Read the model definition and answer for the solid it produces. Units are mm, in the model's axes. Face numbers are marked on the shaded views. Give positions to 0.01 mm unless a question says otherwise; leave off trailing zeros. Order: outer loops, then holes, each group sorted by start corner. A loop starts at its lowest first (then second) coordinate and runs counter-clockwise, first axis right, second up. Notation, with made-up numbers: (59, 48.5) - (65, 48.5) arc R23 cw to (65, 61.5) - close; hole circle Ø5 at (-20.5, 16.25). An arc over 180 degrees is marked (long way). Answer as CSV lines item,"result". Start each with the question number.
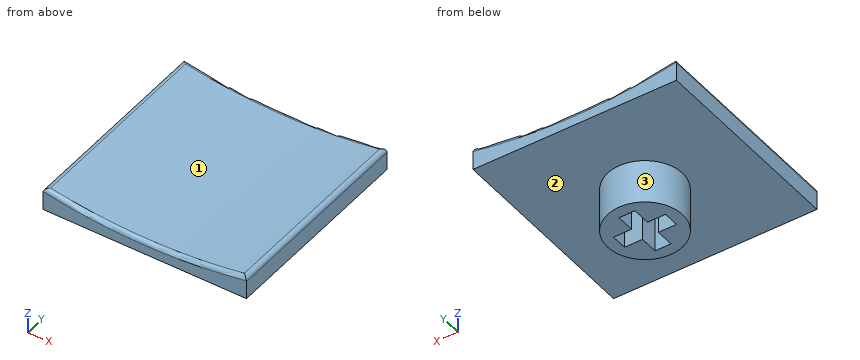
from build123d import *

# Parameters (mm, degrees)
SKETCH_W       = 15.24
SKETCH_H       = 15.24
PAD_DEPTH      = 2
CYLINDER_R     = 40
CYLINDER_DEPTH = 18
FILLET_R       = 0.3
SKETCH001_R    = 2.8
PAD001_DEPTH   = 3.3
POCKET_DEPTH   = 3.3


with BuildPart() as part:
    # Sketch → Pad (new body)
    with BuildSketch(Plane.XY):
        Rectangle(SKETCH_W, SKETCH_H)
    extrude(amount=PAD_DEPTH)

    # Cylinder → Cylinder (cut)
    with BuildSketch(Plane(origin=(0, 9, 41), x_dir=(1, 0, 0), z_dir=(0, -1, 0))):
        Circle(CYLINDER_R)
    extrude(amount=CYLINDER_DEPTH, mode=Mode.SUBTRACT)

    # Fillet
    fillet_edges = [part.edges().sort_by_distance(p)[0] for p in [
        (0, -7.62, 1),
        (-7.62, 0, 1.732512),
        (7.62, 0, 1.732512),
        (0, 7.62, 1),
    ]]
    fillet(fillet_edges, radius=FILLET_R)

    # Sketch001 (on Face4 of Fillet) → Pad001 (join)
    with BuildSketch(Plane(origin=(0, 9, 0), x_dir=(1, 0, 0), z_dir=(0, 0, -1))):
        with Locations((0, 9)):
            Circle(SKETCH001_R)
    extrude(amount=PAD001_DEPTH)

    # Sketch002 (on Face12 of Pad001) → Pocket (cut)
    with BuildSketch(Plane(origin=(0, 9, -3.3), x_dir=(1, 0, 0), z_dir=(0, 0, -1))):
        Polygon((-0.595, 10.95), (0.595, 10.95), (0.595, 9.595), (1.95, 9.595), (1.95, 8.405), (0.595, 8.405), (0.595, 7.05), (-0.595, 7.05), (-0.595, 8.405), (-1.95, 8.405), (-1.95, 9.595), (-0.595, 9.595), align=None)
    extrude(amount=-POCKET_DEPTH, mode=Mode.SUBTRACT)


solid = part.part
(1) Section D-D, the plane y = -5.5 is taken. Write down the section's boundary in (x, z), and give its area (3 significant figures).
(2) Section B-B, the plane x = 0 is taken. Write down the section's boundary in (y, z).
(3) Flat-ended cylindrical pins translate along their axes: pin 1 Ø1.1 at (y, z) = (-1.5, -2.5) entering from +X; pin 2 Ø0.6 at (y, z) = (-0.5, -2) entering from +X; pin 3 Ø2 at (x, y) = (-3.5, 6) entering from -Z. Find the tip coordinate at first contact, or state that the pin passes through.
(4) Section A-A, the plane z = -0.4 is taken. Write down the section's boundary in (x, y) (3 decimals), and give its area (3 significant figures).
(5) Determine the mould class of the marked faces 1, 2 and 3 for opening direction X: released by +X, released by -X, zero draft, split by the parting line, or undercut.
(6) Straight lines are drawn through the part: line 1 (X direction, y = 0.5, z = -2.4) (3 decimals); line 2 (X direction, y = 1.25, z = -1.8) (1 decimal); line 3 (Z direction, x = 4.5, y = 6.75). For each, find the intervals that lie inside material, in ascending order. Write a range as [from, to].
(7) Section C-C, the plane y = 0 is taken. Write down the section's boundary in (x, z).
Checks:
1,outline,"(-7.62, 0) - (7.62, 0) - (7.62, 1.37) arc R0.3 ccw to (7.27, 1.67) arc R40 cw to (-7.27, 1.67) arc R0.3 ccw to (-7.62, 1.37) - close"
1,area,"18.9 mm²"
2,outline,"(-7.62, 0) - (-2.8, 0) - (-2.8, -3.3) - (-1.95, -3.3) - (-1.95, 0) - (1.95, 0) - (1.95, -3.3) - (2.8, -3.3) - (2.8, 0) - (7.62, 0) - (7.62, 0.7) arc R0.3 ccw to (7.32, 1) - (-7.32, 1) arc R0.3 ccw to (-7.62, 0.7) - close"
3,pin 1,"stops at x = 2.63"
3,pin 2,"stops at x = 2.79"
3,pin 3,"stops at z = 0"
4,outline,"circle Ø5.6 at (0, 0); hole (-1.95, -0.595) - (-0.595, -0.595) - (-0.595, -1.95) - (0.595, -1.95) - (0.595, -0.595) - (1.95, -0.595) - (1.95, 0.595) - (0.595, 0.595) - (0.595, 1.95) - (-0.595, 1.95) - (-0.595, 0.595) - (-1.95, 0.595) - close"
4,area,"16.8 mm²"
5,face 1,"undercut"
5,face 2,"zero draft"
5,face 3,"split by the parting line"
6,line 1,"x = [-2.755, -1.95], [1.95, 2.755]"
6,line 2,"x = [-2.5, -0.6], [0.6, 2.5]"
6,line 3,"z = [0, 1.25]"
7,outline,"(-7.62, 0) - (-2.8, 0) - (-2.8, -3.3) - (-1.95, -3.3) - (-1.95, 0) - (1.95, 0) - (1.95, -3.3) - (2.8, -3.3) - (2.8, 0) - (7.62, 0) - (7.62, 1.37) arc R0.3 ccw to (7.27, 1.67) arc R40 cw to (-7.27, 1.67) arc R0.3 ccw to (-7.62, 1.37) - close"
